```python
from build123d import *

# Parameters (mm, degrees)
SKETCH_1_R          = 2.5
EXTRUDE_1_DEPTH     = 3
SKETCH_2_R          = 1.5
EXTRUDE_2_DEPTH     = 25
CUT_EXTRUDE_1_DEPTH = 1.65


with BuildPart() as part:
    # 草图1 → 凸台-拉伸1 (new body)
    with BuildSketch(Plane(origin=(0, 0, 0), x_dir=(1, 0, 0), z_dir=(0, 1, 0))):
        Circle(SKETCH_1_R)
    extrude(amount=EXTRUDE_1_DEPTH)

    # 草图2 → 凸台-拉伸2 (add)
    with BuildSketch(Plane(origin=(0, 3, 0), x_dir=(1, 0, 0), z_dir=(0, 1, 0))):
        Circle(SKETCH_2_R)
    extrude(amount=EXTRUDE_2_DEPTH)

    # 草图3 → 切除-拉伸1 (cut)
    with BuildSketch(Plane.XZ):
        Polygon((1.425, 0), (0.7125, 1.2340862), (-0.7125, 1.2340862), (-1.425, 0), (-0.7125, -1.2340862), (0.7125, -1.2340862), align=None)
    extrude(amount=-CUT_EXTRUDE_1_DEPTH, mode=Mode.SUBTRACT)


solid = part.part
```
Build history of the part. All positions in model axes, mm. A direction names the side the tool comes from. Give positions to 0.01 mm unless a question says otherwise; leave off trailing zeros. Loops run counter-clockwise (first coordinate to the right, second up) from the corner with the lowest first, then second, coordinate; pieces in that order, holes last. Notation, with made-up numbers: (-27.5, -6.5) -> (22.5, -6.5) arc R16 ccw to (22.5, 5.5) -> close; hole circle Ø1 at (-3.75, 57). An arc over 180 degrees is marked (long way). One line per question, with ' | ' between items. Start each with the question number.
1) Cut at D-D (z = -1.85). Give the cut face in (x, y).
2) Cut at A-A (x = 0). Give the cut face in (y, z), plus the area to 3 significant figures.
3) Pin check, flat tip, straight feed: pin 1 (2 mm diameter, centred on y = 9.5, z = -2, fed in from -X). Stop position of the tip, or through.
4) Probe L1, parallel to Y at x = -1.25, z = 1.5; L2, parallel to Y at x = 0.25, z = 0.2; L3, parallel to X at y = 3.5, z = 1.35. List the from-to ranges inside material, lowest first.
5) Cut at C-C (y = 24). Give the cut face in (x, z).
6) Cut at B-B (z = 0.35). Give the cut face in (x, y), plus the area to 3 significant figures.
7) 3-axis set-ups, long thin cutter, end or side, ignore diameter. For faces 1 (the flat face through (0, 3, 2)), 2 (the flat face through (-1.06, 0.81, 0.63)), 3 (the flat face through (0, 28, 0)): which of +Z, -Z, +X, -X, +Y, -Y reach the whole face in a straight line?
8) Two-plate mould, pull along Z, no slides. Class faces 4 (the flat face through (0, 1, 1.234)), 5 (the flat face through (1.1, 0, 1.1)), 6 (the cylindrical face through (-1.5, 15.32, -0.07)): released by +Z, released by -Z, zero draft, split by the parting line, or undercut.
Return value:
1) outline: (-1.68, 0) -> (1.68, 0) -> (1.68, 3) -> (-1.68, 3) -> close
2) outline: (0, -2.5) -> (3, -2.5) -> (3, -1.5) -> (28, -1.5) -> (28, 1.5) -> (3, 1.5) -> (3, 2.5) -> (0, 2.5) -> (0, 1.23) -> (1.65, 1.23) -> (1.65, -1.23) -> (0, -1.23) -> close | area: 85.9 mm^2
3) pin 1: x = -1.12
4) L1: 0 to 3 | L2: 1.65 to 28 | L3: -0.65 to 0.65
5) outline: circle Ø3 at (0, 0)
6) outline: (-2.48, 0) -> (-1.22, 0) -> (-1.22, 1.65) -> (1.22, 1.65) -> (1.22, 0) -> (2.48, 0) -> (2.48, 3) -> (1.46, 3) -> (1.46, 28) -> (-1.46, 28) -> (-1.46, 3) -> (-2.48, 3) -> close | area: 83.7 mm^2
7) face 1: +Y | face 2: -Y | face 3: +Z, -Z, +X, -X, +Y
8) face 4: undercut | face 5: zero draft | face 6: split by the parting line
